```python
from build123d import *

# Parameters (mm, degrees)
F0_W     = 533.4
F0_H     = 88.9
F1_DEPTH = 12.7
F2_W     = 12.7
F2_H     = 12.7
F3_DEPTH = 25.4
F4_W     = 12.7
F4_H     = 12.7
F4_H_2   = 25.4
F5_DEPTH = 25.4
F6_W     = 12.7
F6_H     = 12.7
F7_DEPTH = 25.4


with BuildPart() as f1:
    # F0 (on Top) → F1 (new body)
    with BuildSketch(Plane.XY):
        with Locations((266.7, 44.45)):
            Rectangle(F0_W, F0_H)
    extrude(amount=F1_DEPTH)

    # F2 (on face) → F3 (cut)
    with BuildSketch(Plane.XY.offset(12.7)):
        with Locations((527.05, 6.35)):
            Rectangle(F2_W, F2_H)
        with Locations((527.05, 31.75)):
            Rectangle(F2_W, F2_H)
        with Locations((527.05, 57.15)):
            Rectangle(F2_W, F2_H)
        with Locations((527.05, 82.55)):
            Rectangle(F2_W, F2_H)
    extrude(amount=-F3_DEPTH, mode=Mode.SUBTRACT)

    # F4 (on face) → F5 (cut)
    with BuildSketch(Plane.XY.offset(12.7)):
        with Locations((6.35, 44.45)):
            Rectangle(F4_W, F4_H)
        with Locations((6.35, 69.85)):
            Rectangle(F4_W, F4_H)
        with Locations((6.35, 12.7)):
            Rectangle(F4_W, F4_H_2)
    extrude(amount=-F5_DEPTH, mode=Mode.SUBTRACT)

    # F6 (on face) → F7 (cut)
    with BuildSketch(Plane.XY.offset(12.7)):
        with Locations((19.05, 6.35)):
            Rectangle(F6_W, F6_H)
        with Locations((44.45, 6.35)):
            Rectangle(F6_W, F6_H)
        with Locations((69.85, 6.35)):
            Rectangle(F6_W, F6_H)
        with Locations((95.25, 6.35)):
            Rectangle(F6_W, F6_H)
        with Locations((120.65, 6.35)):
            Rectangle(F6_W, F6_H)
        with Locations((146.05, 6.35)):
            Rectangle(F6_W, F6_H)
        with Locations((171.45, 6.35)):
            Rectangle(F6_W, F6_H)
        with Locations((196.85, 6.35)):
            Rectangle(F6_W, F6_H)
        with Locations((222.25, 6.35)):
            Rectangle(F6_W, F6_H)
        with Locations((247.65, 6.35)):
            Rectangle(F6_W, F6_H)
        with Locations((273.05, 6.35)):
            Rectangle(F6_W, F6_H)
        with Locations((298.45, 6.35)):
            Rectangle(F6_W, F6_H)
        with Locations((323.85, 6.35)):
            Rectangle(F6_W, F6_H)
        with Locations((349.25, 6.35)):
            Rectangle(F6_W, F6_H)
        with Locations((374.65, 6.35)):
            Rectangle(F6_W, F6_H)
        with Locations((400.05, 6.35)):
            Rectangle(F6_W, F6_H)
        with Locations((425.45, 6.35)):
            Rectangle(F6_W, F6_H)
        with Locations((450.85, 6.35)):
            Rectangle(F6_W, F6_H)
        with Locations((476.25, 6.35)):
            Rectangle(F6_W, F6_H)
        with Locations((501.65, 6.35)):
            Rectangle(F6_W, F6_H)
    extrude(amount=-F7_DEPTH, mode=Mode.SUBTRACT)


solid = f1.part
```
Input: part model. Units: mm. Frame: model coordinates. A direction names the side the tool comes from. Coordinates: 2 decimals unless noted, no trailing zeros. Loops run counter-clockwise (first coordinate to the right, second up) from the corner with the lowest first, then second, coordinate; pieces in that order, holes last. Notation, with made-up numbers: M -31.5,13.25 L -5.5,13.25 A23 ccw -5.5,24.25 Z; hole C -36.5,71 d11. An arc over 180 degrees is marked long. Use a Markdown table: item, result. Add a question column.
1) Set-up query: faces 4 (the flat face through (121, 12.7, 6)), 5 (the flat face through (12.7, 70, 6)), 6 (the flat face through (520.7, 82, 6)), 7 (the flat face through (25.4, 6, 6)), 8 (the flat face through (527, 38.1, 6)). Return all of +Z, -Z, +X, -X, +Y, -Y with unobstructed straight access to the full face (end or side cutting, diameter ignored); none if empty.
2) Pin query (flat end, axial travel): P1, Ø6.5, axis at x = 169, z = 6.5, coming from the -Y side; P2, Ø4, axis at y = 8, z = 6.5, coming from the +X side; P3, Ø6.5, axis at y = 4, z = 8.5, coming from the -X side. Return the tip coordinate at first contact, or that it passes through.
3) Draft query along X for faces 1 (the flat face through (495.3, 6, 6)), 2 (the flat face through (527, 76.2, 6)), 3 (the flat face through (520.7, 6, 6)). Return one class per face: +X half, -X half, draft (parallel to the pull), parting line (faces both ways), or undercut.
4) Section A-A, the plane y = 19.5. Return the cut outline in (x, z), plus the area to 3 significant figures.
5) Line query: L1, parallel to X at y = 42.5, z = 9; L2, parallel to Y at x = 126, z = 4.75; L3, parallel to X at y = 27, z = 8.25. Output: solid intervals per line, ascending. Write a range as from..to.
Answer below:
| question | item | result |
|---|---|---|
| 1 | face 4 | +Z, -Z, -Y |
| 1 | face 5 | +Z, -Z, -X |
| 1 | face 6 | +Z, -Z, +X, +Y |
| 1 | face 7 | +Z, -Z, -X, -Y |
| 1 | face 8 | +Z, -Z, +X |
| 2 | P1 | y = 12.7 |
| 2 | P2 | x = 520.7 |
| 2 | P3 | x = 25.4 |
| 3 | face 1 | undercut |
| 3 | face 2 | draft |
| 3 | face 3 | +X half |
| 4 | outline | M 12.7,0 L 533.4,0 L 533.4,12.7 L 12.7,12.7 Z |
| 4 | area | 6,610 mm2 |
| 5 | L1 | 12.7..533.4 |
| 5 | L2 | 12.7..88.9 |
| 5 | L3 | 0..520.7 |
